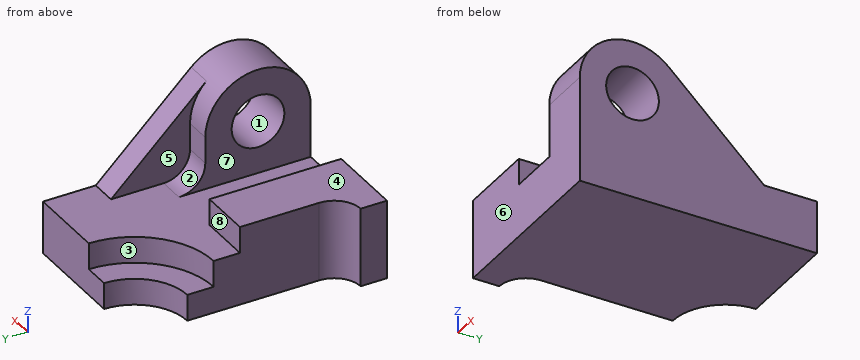
from build123d import *

# Parameters (mm, degrees)
SKETCH1_W           = 6
SKETCH1_H           = 9
BOSS_EXTRUDE1_DEPTH = 2
CUT_EXTRUDE1_DEPTH  = 3
CUT_EXTRUDE2_DEPTH  = 1
SKETCH4_W           = 2
SKETCH4_H           = 5
BOSS_EXTRUDE2_DEPTH = 1
BOSS_EXTRUDE3_DEPTH = 3
SKETCH7_R           = 1
BOSS_EXTRUDE4_DEPTH = 2
BOSS_EXTRUDE5_DEPTH = 1


with BuildPart() as part:
    # Sketch1 → Boss-Extrude1 (new body)
    with BuildSketch(Plane.XY):
        Rectangle(SKETCH1_W, SKETCH1_H)
    extrude(amount=BOSS_EXTRUDE1_DEPTH)

    # Sketch2 → Cut-Extrude1 (cut, through all)
    with BuildSketch(Plane.XY.offset(2)):
        with BuildLine():
            Line((-1, 4.5), (-3, 4.5))
            Line((-3, 4.5), (-3, 2.5))
            ThreePointArc((-3, 2.5), (-1.585786438, 3.085786438), (-1, 4.5))
        make_face()
    extrude(amount=-CUT_EXTRUDE1_DEPTH, mode=Mode.SUBTRACT)

    # Sketch3 → Cut-Extrude2 (cut)
    with BuildSketch(Plane.XY.offset(2)):
        with BuildLine():
            Line((0, 4.5), (-3, 4.5))
            Line((-3, 4.5), (-3, 1.5))
            ThreePointArc((-3, 1.5), (-0.878679656, 2.378679656), (0, 4.5))
        make_face()
    extrude(amount=-CUT_EXTRUDE2_DEPTH, mode=Mode.SUBTRACT)

    # Sketch4 → Boss-Extrude2 (add)
    with BuildSketch(Plane.XY.offset(2)):
        with Locations((-2, -2)):
            Rectangle(SKETCH4_W, SKETCH4_H)
    extrude(amount=BOSS_EXTRUDE2_DEPTH)

    # Sketch5 → Boss-Extrude3 (add)
    with BuildSketch(Plane.XY.offset(3)):
        with BuildLine():
            Line((-3, -4.5), (-4, -4.5))
            Line((-4, -4.5), (-4, -3.5))
            ThreePointArc((-4, -3.5), (-3.292893219, -3.207106781), (-3, -2.5))
            Line((-3, -2.5), (-3, -4.5))
        make_face()
    extrude(amount=-BOSS_EXTRUDE3_DEPTH)

    # Sketch7 → Boss-Extrude4 (add)
    with BuildSketch(Plane(origin=(3, 0, 0), x_dir=(0, 0, -1), z_dir=(1, 0, 0))):
        with BuildLine():
            Line((-4, -4.5), (-2, -4.5))
            Line((-2, -4.5), (-2, 0.5))
            ThreePointArc((-2, 0.5), (-2.292893219, -0.207106781), (-3, -0.5))
            Line((-3, -0.5), (-4, -0.5))
            ThreePointArc((-4, -0.5), (-6, -2.5), (-4, -4.5))
        make_face()
        with Locations((-4, -2.5)):
            Circle(SKETCH7_R, mode=Mode.SUBTRACT)
    extrude(amount=-BOSS_EXTRUDE4_DEPTH)

    # Sketch8 → Boss-Extrude5 (add)
    with BuildSketch(Plane(origin=(3, 0, 0), x_dir=(0, 0, -1), z_dir=(1, 0, 0))):
        with BuildLine():
            Line((-2, 2.5), (-5.448275862, -1.120689655))
            ThreePointArc((-5.448275862, -1.120689655), (-4.787838597, -0.66170994), (-4, -0.5))
            Line((-4, -0.5), (-3, -0.5))
            ThreePointArc((-3, -0.5), (-2.292893219, -0.207106781), (-2, 0.5))
            Line((-2, 0.5), (-2, 2.5))
        make_face()
    extrude(amount=-BOSS_EXTRUDE5_DEPTH)


solid = part.part
For this review, take the finished solid that the model builds, in its own axes (mm). Face numbers are marked on the shaded views. A direction names the side the tool comes from. Give positions to 0.01 mm unless a question says otherwise; leave off trailing zeros. Loops run counter-clockwise (first coordinate to the right, second up) from the corner with the lowest first, then second, coordinate; pieces in that order, holes last.
Item 1: Take a section at C-C, the plane z = 1.3. State the section outline as (x, y) points, and give its area (3 significant figures).
Item 2: Draft analysis for pull direction X (two halves, no side actions). For the marked faces 1, 2 and 3, state which applies: +X half, -X half, draft (parallel to the pull), parting line (faces both ways), or undercut.
Item 3: Take a section at D-D, the plane y = -3. State the section outline as (x, z) points.
Item 4: Take a section at A-A, the plane z = 3.2. State the section outline as (x, y) points, and give its area (3 significant figures).
Item 5: Take a section at B-B, the plane x = 1.5. State the section outline as (y, z) points.
Item 6: For line 1 along Z through (x, y) = (-1.5, -1.5); line 2 along Y through (x, z) = (1.85, 4); line 3 along Z through (x, y) = (1.75, 4), list the stretches that pass through material, from the lowest coordinate up.
Item 7: Insertion check: pin 1 (1.1 mm diameter, centred on x = -2.5, z = 2.5, fed in from +Y); pin 2 (0.9 mm diameter, centred on x = -2.5, y = -1.5, fed in from +Z); pin 3 (1.5 mm diameter, centred on x = -1.5, y = 2.5, fed in from +Z). Each pin has a flat end and moves straight along its axis. Give the tip position at first contact, or say it passes through.
Item 8: Tool access review of the marked faces 4, 5, 6, 7 and 8: name each direction out of +Z, -Z, +X, -X, +Y, -Y from which nothing blocks a thin tool from reaching the whole face with its end or side.
Calculated:
1. outline: (-4, -4.5) - (3, -4.5) - (3, 4.5) - (0, 4.5) arc R3 cw to (-3, 1.5) - (-3, -2.5) arc R1 cw to (-4, -3.5) - close
1. area: 48.1 mm2
2. face 1: draft
2. face 2: undercut
2. face 3: -X half
3. outline: (-3.13, 0) - (3, 0) - (3, 3.13) - (1, 3.13) - (1, 2) - (-1, 2) - (-1, 3) - (-3.13, 3) - close; (1, 4.87) - (3, 4.87) - (3, 5.94) - (1, 5.94) - close
4. outline: (1, -4.5) - (3, -4.5) - (3, -3.1) - (1, -3.1) - close; (1, -1.9) - (3, -1.9) - (3, 1.24) - (2, 1.24) - (2, -0.5) - (1, -0.5) - close
4. area: 7.34 mm2
5. outline: (-4.5, 0) - (4.5, 0) - (4.5, 2) - (0.5, 2) arc R1 cw to (-0.5, 3) - (-0.5, 4) arc R2 ccw to (-4.5, 4) - close; hole circle Ø2 at (-2.5, 4)
6. line 1: z = 0 to 3
6. line 2: y = -4.5 to -3.5, -1.5 to -0.5
6. line 3: z = 0 to 2
7. pin 1: stops at y = 1.59
7. pin 2: stops at z = 3
7. pin 3: stops at z = 2
8. face 4: +Z, -X, +Y, -Y
8. face 5: +Z, +Y
8. face 6: +Z, -Z, +X, -X, -Y
8. face 7: +Z, +Y, -Y
8. face 8: +Z, -X, +Y
